```python
from build123d import *

# Parameters (mm, degrees)
BOSS_EXTRUDE1_DEPTH = 20
BOSS_EXTRUDE2_DEPTH = 20
SWEEP1_START        = 164
SWEEP1_OUTLINE_R    = 5
SWEEP1_DEPTH        = 186
SKETCH4_W           = 100
SKETCH4_H           = 10
BOSS_EXTRUDE3_DEPTH = 50
CUT_EXTRUDE1_DEPTH  = 50
FILLET1_START       = 10
FILLET1_DEPTH       = 10
FILLET1_2_DEPTH     = 10


with BuildPart() as part:
    # Sketch1 → Boss-Extrude1 (new body)
    with BuildSketch(Plane(origin=(0, 0, 0), x_dir=(1, 0, 0), z_dir=(0, 1, 0))):
        with BuildLine():
            Line((-82.5, 142.894191624), (-67.5, 116.913429511))
            ThreePointArc((-67.5, 116.913429511), (67.5, 116.913429511), (135, 0))
            ThreePointArc((135, 0), (131.799960961, -29.219347882), (122.35155125, -57.053465335))
            Line((122.35155125, -57.053465335), (149.540784861, -69.732013187))
            ThreePointArc((149.540784861, -69.732013187), (161.088841175, -35.7125363), (165, 0))
            ThreePointArc((165, 0), (82.5, 142.894191624), (-82.5, 142.894191624))
        make_face()
    extrude(amount=BOSS_EXTRUDE1_DEPTH)

    # Sketch2 → Boss-Extrude2 (add)
    with BuildSketch(Plane(origin=(0, 20, 0), x_dir=(1, 0, 0), z_dir=(0, 1, 0))):
        with BuildLine():
            ThreePointArc((122.35155125, -57.053465335), (91.204678028, 99.532440469), (-67.5, 116.913429511))
            Line((-67.5, 116.913429511), (-57.5, 99.592921435))
            ThreePointArc((-57.5, 99.592921435), (57.5, 99.592921435), (115, 0))
            ThreePointArc((115, 0), (112.274040819, -24.890555603), (104.225395509, -48.6011001))
            Line((104.225395509, -48.6011001), (122.35155125, -57.053465335))
        make_face()
        with BuildLine():
            Line((-82.5, 142.894191624), (-67.5, 116.913429511))
            ThreePointArc((-67.5, 116.913429511), (91.204678028, 99.532440469), (122.35155125, -57.053465335))
            Line((122.35155125, -57.053465335), (149.540784861, -69.732013187))
            ThreePointArc((149.540784861, -69.732013187), (111.472384257, 121.650760574), (-82.5, 142.894191624))
        make_face()
    extrude(amount=BOSS_EXTRUDE2_DEPTH)

    # Sweep1: read off the stored shape, not the designer's step
    # Sweep1 outline → Sweep1 (add)
    with BuildSketch(Plane.YZ.offset(SWEEP1_START)):
        with Locations((15, 0)):
            Circle(SWEEP1_OUTLINE_R)
    extrude(amount=SWEEP1_DEPTH)

    # Sketch4 → Boss-Extrude3 (add)
    with BuildSketch(Plane(origin=(350, 0, 0), x_dir=(1.4081184135372707e-12, 0, -1.0), z_dir=(1.0, 0, 1.4081184135372707e-12))):
        with Locations((0, 15)):
            Rectangle(SKETCH4_W, SKETCH4_H)
    extrude(amount=BOSS_EXTRUDE3_DEPTH)

    # Sketch5 → Cut-Extrude1 (cut)
    with BuildSketch(Plane(origin=(0, 20, 0), x_dir=(1, 0, 0), z_dir=(0, 1, 0))):
        Polygon((360, 40), (360, 0), (360, -40), (390, -40), (390, 40), align=None)
    extrude(amount=-CUT_EXTRUDE1_DEPTH, mode=Mode.SUBTRACT)

    # Fillet1: read off the stored shape, not the designer's step
    # Fillet1 outline → Fillet1 (cut)
    with BuildSketch(Plane(origin=(0, 0, 0), x_dir=(1, 0, 0), z_dir=(0, 1, 0)).offset(FILLET1_START)):
        with BuildLine():
            ThreePointArc((390, 50), (397.071067812, 47.071067812), (400, 40))
            Line((400, 40), (400, 50))
            Line((400, 50), (390, 50))
        make_face()
        with BuildLine():
            Line((400, -50), (400, -40))
            ThreePointArc((400, -40), (397.071067812, -47.071067812), (390, -50))
            Line((390, -50), (400, -50))
        make_face()
        with BuildLine():
            ThreePointArc((350, 40), (352.928932188, 47.071067812), (360, 50))
            Line((360, 50), (350, 50))
            Line((350, 50), (350, 40))
        make_face()
        with BuildLine():
            Line((350, -50), (360, -50))
            ThreePointArc((360, -50), (352.928932188, -47.071067812), (350, -40))
            Line((350, -40), (350, -50))
        make_face()
    extrude(amount=FILLET1_DEPTH, mode=Mode.SUBTRACT)

    # Fillet1 2 outline → Fillet1 2 (add)
    with BuildSketch(Plane(origin=(0, 0, 0), x_dir=(1, 0, 0), z_dir=(0, 1, 0)).offset(FILLET1_START)):
        with BuildLine():
            Line((390, -40), (390, -30))
            ThreePointArc((390, -30), (387.071067812, -37.071067812), (380, -40))
            Line((380, -40), (390, -40))
        make_face()
        with BuildLine():
            ThreePointArc((380, 40), (387.071067812, 37.071067812), (390, 30))
            Line((390, 30), (390, 40))
            Line((390, 40), (380, 40))
        make_face()
        with BuildLine():
            Line((360, -40), (370, -40))
            ThreePointArc((370, -40), (362.928932188, -37.071067812), (360, -30))
            Line((360, -30), (360, -40))
        make_face()
        with BuildLine():
            ThreePointArc((360, 30), (362.928932188, 37.071067812), (370, 40))
            Line((370, 40), (360, 40))
            Line((360, 40), (360, 30))
        make_face()
    extrude(amount=FILLET1_2_DEPTH)


solid = part.part
```
CAD build for the part. Positions are in the model's coordinates, mm. A direction names the side the tool comes from. Round coordinates to 2 decimals unless told otherwise and drop trailing zeros. Write each loop counter-clockwise with the first axis right and the second up, starting at its lowest first coordinate (ties: lowest second). Pieces come first, ordered by that corner, then holes. Notation, with made-up numbers: (46.5, 88) - (71.5, 88) arc R32 ccw to (71.5, 118) - close; hole circle Ø1 at (26, -2.5). An arc over 180 degrees is marked (long way). Write item = value, one per line. Start each with the question number.
Q1. Band-saw the part on B-B (z = 14.5). Give the cut face in (x, y).
Q2. Band-saw the part on D-D (x = 141). Give the cut face in (y, z).
Q3. Band-saw the part on A-A (y = 15). Give the cut face in (x, z), then the cut area to 3 significant figures.
Q4. Probe L1, parallel to X at y = 2, z = 2.5; L2, parallel to Z at x = 378, y = 17; L3, parallel to X at y = 15, z = 25 (3 decimals). List the from-to ranges inside material, lowest first. Write a range as from..to.
Q5. Drop flat-ended pins along their axis: pin 1 (10 mm diameter, centred on x = 289.5, y = 22, fed in from -Z); pin 2 (3 mm diameter, centred on y = 13.5, z = 26, fed in from -X); pin 3 (4 mm diameter, centred on y = 25, z = -89.5, fed in from -X); pin 4 (15 mm diameter, centred on x = 376.5, z = 11.5, fed in from +Y). Give the stop position or say it passes through.
Q6. Which spindle directions (+Z, -Z, +X, -X, +Y, -Y) get a long thin tool onto all of the face, cutting with end or side? Do faces 4 (the flat face through (86, 20, -82)), 5 (the cylindrical face through (386.99, 14.93, -37.15)), 6 (the flat face through (375, 15, 50)), 7 (the flat face through (375, 15, -50)). Say none if no direction does.
Q7. Band-saw the part on C-C (x = 292). Give the cut face in (y, z).
Q8. Mould opens along Z. For faces 1 (the flat face through (375, 15, 40)), 2 (the cylindrical face through (352.85, 14.93, -46.99)), 3 (the cylindrical face through (353.01, 14.93, 47.15)) say: pulls with the +Z half, pulls with the -Z half, needs draft (parallel to the pull), parting line crosses it, or undercut.
Answers below:
q1.outline = (114.08, 20) - (134.22, 20) - (134.22, 0) - (164.36, 0) - (164.36, 40) - (114.08, 40) - close; (350, 10) - (360, 10) - (360, 20) - (350, 20) - close; (390, 10) - (400, 10) - (400, 20) - (390, 20) - close
q2.outline = (0, -85.7) - (40, -85.7) - (40, 65.75) - (0, 65.75) - close
q3.outline = (-82.5, -142.89) arc R165 ccw to (164.92, -5) - (350, -5) - (350, -40) arc R10 ccw to (360, -50) - (390, -50) arc R10 ccw to (400, -40) - (400, 40) arc R10 ccw to (390, 50) - (360, 50) arc R10 ccw to (350, 40) - (350, 5) - (164.92, 5) arc R165 ccw to (149.54, 69.73) - (122.35, 57.05) arc R135 cw to (-67.5, -116.91) - close; hole (360, -30) arc R10 ccw to (370, -40) - (380, -40) arc R10 ccw to (390, -30) - (390, 30) arc R10 ccw to (380, 40) - (370, 40) arc R10 ccw to (360, 30) - close
q3.area = 15,800 mm2
q4.L1 = 134.98..164.98
q4.L2 = -50..-40, 40..50
q4.L3 = 132.665..163.095, 350..360, 390..400
q5.pin_1 = -4.58
q5.pin_2 = 132.17
q5.pin_3 = 69.66
q5.pin_4 = through
q6.face_4 = -Y
q6.face_5 = +Y, -Y
q6.face_6 = +Z, +X, +Y, -Y
q6.face_7 = -Z, +X, +Y, -Y
q7.outline = circle Ø10 at (15, 0)
q8.face_1 = undercut
q8.face_2 = pulls with the -Z half
q8.face_3 = pulls with the +Z half
